from build123d import *

# Parameters (mm, degrees)
BOSS_EXTRUDE1_DEPTH     = 18.5
CUT_EXTRUDE3_START      = -10
CUT_EXTRUDE3_DEPTH      = 10
SKETCH4_R               = 5
CUT_EXTRUDE4_DEPTH      = 53.156015952
SKETCH5_R               = 12
CUT_EXTRUDE5_DEPTH      = 37
SKETCH6_R               = 3
CUT_EXTRUDE6_DEPTH      = 13
CUT_EXTRUDE7_REACH      = 52.52
CUT_EXTRUDE7_END_RADIUS = 19
SKETCH7_R               = 2


# Read off the part's stored shape, not the designer's step: Cut-Extrude3
with BuildPart() as part:
    # Sketch2 → Boss-Extrude1 (new, symmetric)
    with BuildSketch(Plane.XY):
        with BuildLine():
            Line((-18.027756377, 6), (-22, 6))
            Line((-22, 6), (-22, 19))
            Line((-22, 19), (-43, 19))
            Line((-43, 19), (-43, 29))
            Line((-43, 29), (-24.556058316, 29))
            ThreePointArc((-24.556058316, 29), (0, 38), (24.556058316, 29))
            Line((24.556058316, 29), (43, 29))
            Line((43, 29), (43, 19))
            Line((43, 19), (22, 19))
            Line((22, 19), (22, 6))
            Line((22, 6), (18.027756377, 6))
            ThreePointArc((18.027756377, 6), (0, 19), (-18.027756377, 6))
        make_face()
    extrude(amount=BOSS_EXTRUDE1_DEPTH, both=True)

    # Cut-Extrude3 outline → Cut-Extrude3 (cut)
    with BuildSketch(Plane(origin=(0, 29, 0), x_dir=(1, 0, 0), z_dir=(0, 1, 0)).offset(CUT_EXTRUDE3_START)):
        with BuildLine():
            ThreePointArc((43, 0), (41.941183485, -9.483518751), (38.816877772, -18.5))
            Line((38.816877772, -18.5), (43, -18.5))
            Line((43, -18.5), (43, 0))
        make_face()
        with BuildLine():
            ThreePointArc((38.816877772, 18.5), (41.941183485, 9.483518751), (43, 0))
            Line((43, 0), (43, 18.5))
            Line((43, 18.5), (38.816877772, 18.5))
        make_face()
        with BuildLine():
            Line((-43, -18.5), (-38.816877772, -18.5))
            ThreePointArc((-38.816877772, -18.5), (-41.941183485, -9.483518751), (-43, 0))
            Line((-43, 0), (-43, -18.5))
        make_face()
        with BuildLine():
            Line((-43, 18.5), (-43, 0))
            ThreePointArc((-43, 0), (-41.941183485, 9.483518751), (-38.816877772, 18.5))
            Line((-38.816877772, 18.5), (-43, 18.5))
        make_face()
    extrude(amount=CUT_EXTRUDE3_DEPTH, mode=Mode.SUBTRACT)

    # Sketch4 → Cut-Extrude4 (cut, through all)
    with BuildSketch(Plane(origin=(0, 29, 0), x_dir=(1, 0, 0), z_dir=(0, 1, 0))):
        with Locations(Location((-31, 0, 0), (0, 0, 270))):
            Circle(SKETCH4_R)
        with Locations(Location((31, 0, 0), (0, 0, 180))):
            Circle(SKETCH4_R)
    extrude(amount=-CUT_EXTRUDE4_DEPTH, mode=Mode.SUBTRACT)

    # Sketch5 → Cut-Extrude5 (cut)
    with BuildSketch(Plane(origin=(0, 29, 0), x_dir=(1, 0, 0), z_dir=(0, 1, 0))):
        with Locations((-31, 0)):
            Circle(SKETCH5_R)
        with Locations((31, 0)):
            Circle(SKETCH5_R)
    extrude(amount=CUT_EXTRUDE5_DEPTH, mode=Mode.SUBTRACT)

    # Sketch6 → Cut-Extrude6 (cut)
    with BuildSketch(Plane(origin=(0, 38, 0), x_dir=(1, 0, 0), z_dir=(0, 1, 0))):
        with Locations(Location((0, 0, 0), (0, 0, 270))):
            Circle(SKETCH6_R)
    extrude(amount=-CUT_EXTRUDE6_DEPTH, mode=Mode.SUBTRACT)

    # Cut-Extrude7: up to this cylinder (the profile starts outside it)
    cut_extrude7_end = Plane(origin=(0, 0, 0), z_dir=(0, 0, -1)) * Cylinder(CUT_EXTRUDE7_END_RADIUS, 144.04, mode=Mode.PRIVATE)
    # Sketch7 → Cut-Extrude7 (cut, up to the surface)
    with BuildSketch(Plane(origin=(0, 25, 0), x_dir=(1, 0, 0), z_dir=(0, 1, 0)), mode=Mode.PRIVATE) as cut_extrude7_sk1:
        with Locations(Location((0, 0, 0), (0, 0, 270))):
            Circle(SKETCH7_R)
    cut_extrude7_tool1 = extrude(cut_extrude7_sk1.sketch, amount=-CUT_EXTRUDE7_REACH, mode=Mode.PRIVATE) - cut_extrude7_end
    add(cut_extrude7_tool1.solids().sort_by_distance((0, 25, 0))[0], mode=Mode.SUBTRACT)


solid = part.part
Input: part model. Units: mm. Frame: model coordinates. A direction names the side the tool comes from. Round coordinates to 2 decimals unless told otherwise and drop trailing zeros. Write each loop counter-clockwise with the first axis right and the second up, starting at its lowest first coordinate (ties: lowest second). Pieces come first, ordered by that corner, then holes.
1) Contact query for flat-ended pins moving along their axis: P1, Ø16, axis at x = -31, z = 0, coming from the +Y side; P2, Ø4, axis at x = -11, z = -7, coming from the -Y side; P3, Ø1.5, axis at y = 17, z = 10, coming from the -X side; P4, Ø6.5, axis at x = 0, z = 0, coming from the +Y side. Output: stop coordinate, or through.
2) Draft query along X for faces 5 (the flat face through (-35, 19, 4)), 6 (the cylindrical face through (36, 24, 0)), 7 (the flat face through (-22, 12, 0)). Return one class per face: pulls with the +X half, pulls with the -X half, needs draft (parallel to the pull), parting line crosses it, or undercut.
3) Reachability of faces 1 (the flat face through (-33.8, 29, 4.4)), 2 (the cylindrical face through (3, 32, 0)), 3 (the cylindrical face through (19, 30, 0)), 4 (the flat face through (22, 13, 0)) from +Z, -Z, +X, -X, +Y, -Y: full face, straight path, thin tool, end or side. Return the list, or none.
4) Ray query, L1, parallel to Z at x = 31, y = 23.5; L2, parallel to Z at x = 0, y = 32.25; L3, parallel to Y at x = 29.5, z = -7.5. Return the intervals inside material, ascending.
5) Cut plane A-A (x = -31). Return the cut outline in (y, z).
6) Cut plane C-C (z = 8.5). Return the cut outline in (x, y).
7) Cut plane D-D (y = 30). Return the cut outline in (x, z).
8) Cut plane B-B (y = 22). Return the cut outline in (x, z).
Geometry says:
1. P1: stops at y = 29
1. P2: stops at y = 13.86
1. P3: stops at x = -22
1. P4: stops at y = 38
2. face 5: needs draft
2. face 6: undercut
2. face 7: pulls with the -X half
3. face 1: -X, +Y
3. face 2: +Y
3. face 3: +X, +Y
3. face 4: +Z, -Z, +X, -Y
4. L1: z = -18.5 to -5, 5 to 18.5
4. L2: z = -18.5 to -3, 3 to 18.5
4. L3: y = 19 to 29
5. outline: (19, -18.5) - (29, -18.5) - (29, -5) - (19, -5) - close; (19, 5) - (29, 5) - (29, 18.5) - (19, 18.5) - close
6. outline: (-42.15, 19) - (-22, 19) - (-22, 6) - (-18.03, 6) arc R19 cw to (18.03, 6) - (22, 6) - (22, 19) - (42.15, 19) - (42.15, 29) - (22.53, 29) - (22.53, 30.6) arc R38 ccw to (-22.53, 30.6) - (-22.53, 29) - (-42.15, 29) - close
7. outline: (-23.32, -18.5) - (23.32, -18.5) - (23.32, -9.22) arc R12 cw to (23.32, 9.22) - (23.32, 18.5) - (-23.32, 18.5) - (-23.32, 9.22) arc R12 cw to (-23.32, -9.22) - close; hole circle Ø6 at (0, 0)
8. outline: (-38.82, -18.5) - (38.82, -18.5) arc R43 ccw to (38.82, 18.5) - (-38.82, 18.5) arc R43 ccw to start; hole circle Ø10 at (-31, 0); hole circle Ø4 at (0, 0); hole circle Ø10 at (31, 0)
